The drawing under review shows one solid part. Ordinate dimensions are in mm from its lowest x, y, z. Coordinates: 2 decimals unless noted, no trailing zeros. Answer as CSV lines item,"result". Start each with the question number.
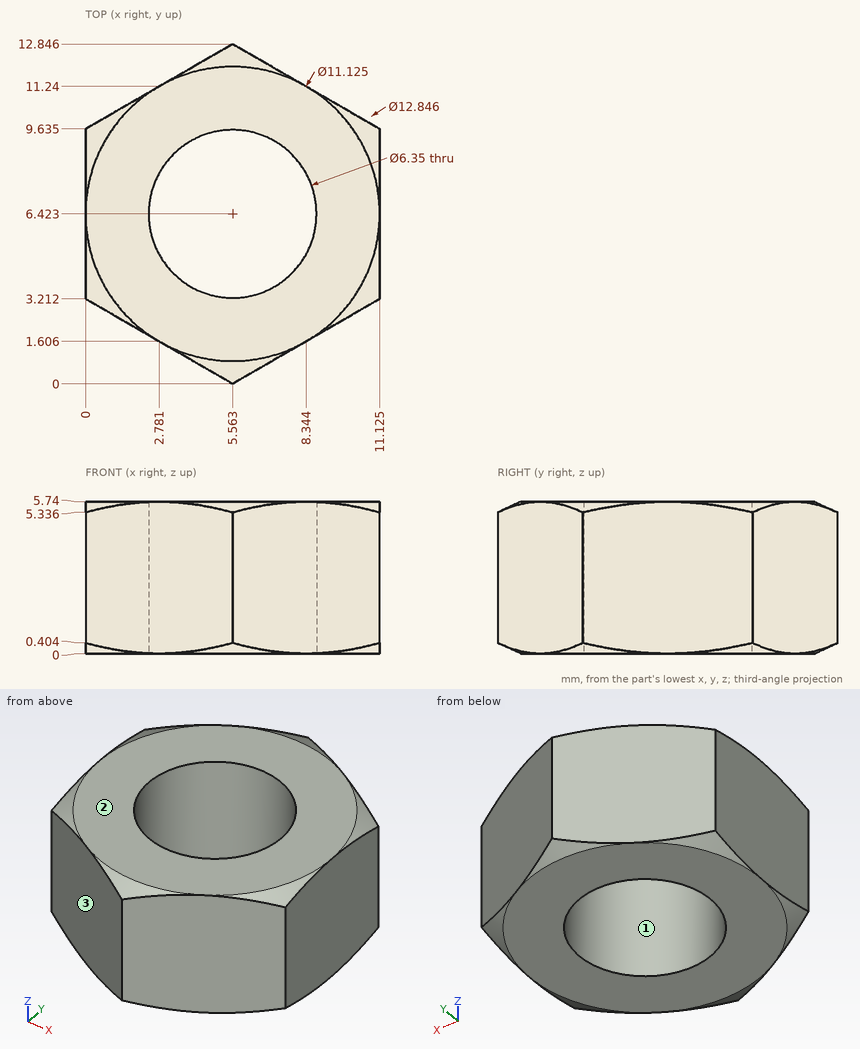
1) Mouldability with a two-part tool opening along Y and no side actions: class the marked faces 1, 2 and 3 as +Y half, -Y half, draft (parallel to the pull), parting line (faces both ways), or undercut.
2) To check wall thickness, follow line 1 (Y direction, x = 7.25, z = 0.2) (1 decimal); line 2 (X direction, y = 4.5, z = 0.8) (1 decimal); line 3 (Y direction, x = 8, z = 5.25) (1 decimal). State the ranges of each line that lie inside material, in increasing order. Write a range as [from, to].
3) Clearance check with a flat-ended pin moving along its axis: pin 1 Ø1.5 at (x, z) = (4.5, 4) entering from -Y. State where the tip first meets the part, or that it passes through.
Results:
1,face 1,"undercut"
1,face 2,"draft"
1,face 3,"-Y half"
2,line 1,"y = [1, 3.7], [9.1, 11.9]"
2,line 2,"x = [0, 3], [8.1, 11.1]"
2,line 3,"y = [1.4, 4.4], [8.5, 11.4]"
3,pin 1,"stops at y = 0.18"
